The figure shows three views and two pictorial views of one solid part (mm, origin at its lowest corner). Answer the questions. A direction names the side the tool comes from. Round coordinates to 2 decimals unless told otherwise and drop trailing zeros. Order: outer loops, then holes, each group sorted by start corner. A loop starts at its lowest first (then second) coordinate and runs counter-clockwise, first axis right, second up. Notation, with made-up numbers: (36, 68) - (50, 68) arc R15 cw to (50, 94) - close; hole circle Ø8 at (-33, -4.5). An arc over 180 degrees is marked (long way). Use CSV: the item, a comma, the result in double quotes. Start each with the question number.
Item 1: For the marked faces 5, 6 and 7, determine the directions among +Z, -Z, +X, -X, +Y, -Y from which every point of the face is accessible in a straight line to the end or side of a thin tool.
Item 2: Find section D-D, the plane z = 3. Give the vertices of the cut face in (x, y), plus the area to 3 significant figures.
Item 3: Find section A-A, the plane z = 13. Give the vertices of the cut face in (x, y).
Item 4: Straight lines are drawn through the part: line 1 along X through (y, z) = (2.65, 13); line 2 along Z through (x, y) = (10, 1.55); line 3 along X through (y, z) = (3, 7). For each, find the intervals that lie inside material, in ascending order. Write a range as [from, to].
Item 5: Find section C-C, the plane y = 6. Give the vertices of the cut face in (x, z).
Item 6: Flat-ended cylindrical pins translate along their axes: P1, Ø8, axis at x = 32, y = 37.5, coming from the +Z side; P2, Ø1.5, axis at y = 31, z = 10, coming from the +X side; P3, Ø6, axis at x = 20.5, z = 7.5, coming from the +Y side (1 decimal); P4, Ø1.8, axis at x = 4, z = 13, coming from the -Y side. Find the tip coordinate at first contact, or state that the pin passes through.
Item 7: Determine the mould class of the marked faces 1, 2, 3 and 4 for opening direction Y: +Y half, -Y half, draft (parallel to the pull), parting line (faces both ways), or undercut.
Item 8: Find section B-B, the plane x = 10. Give the vertices of the cut face in (y, z).
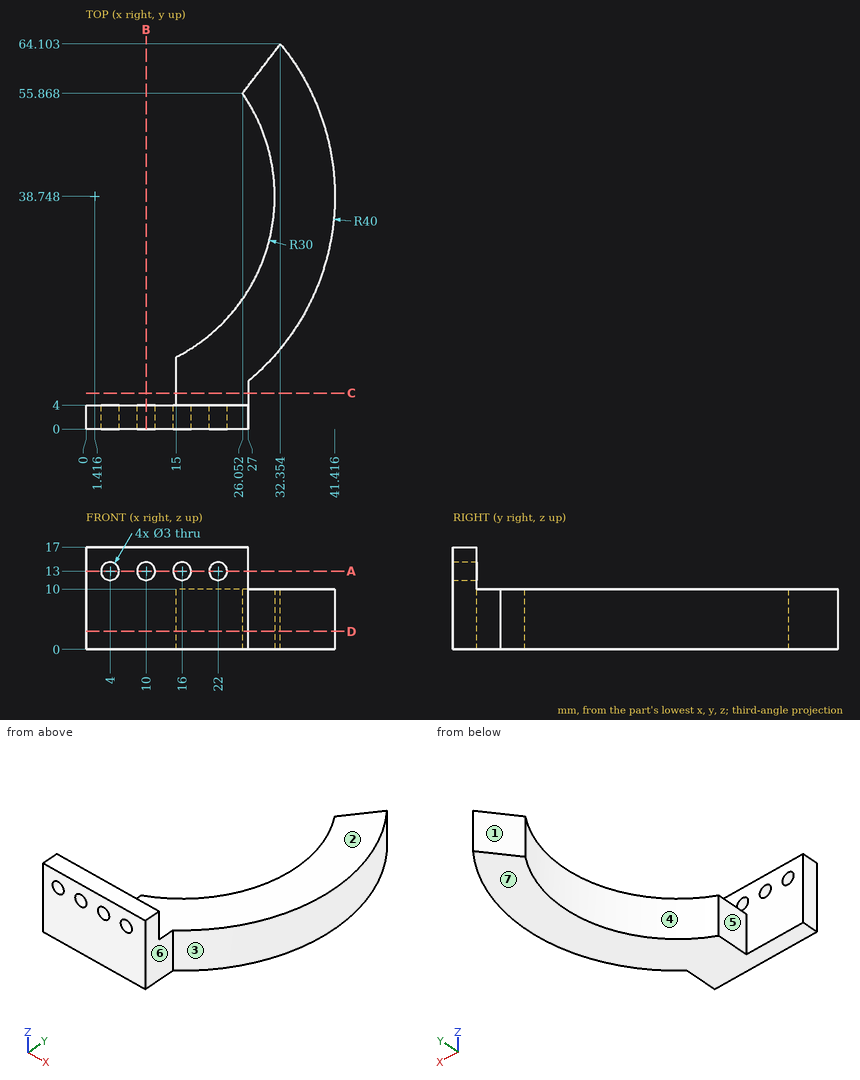
Worked out:
1,face 5,"+Z, -Z, -X, +Y"
1,face 6,"+Z, -Z, +X, -Y"
1,face 7,"-Z, +X, -X, +Y, -Y"
2,outline,"(0, 0) - (27, 0) - (27, 8) arc R40 ccw to (32.35, 64.1) - (26.05, 55.87) arc R30 cw to (15, 12) - (15, 4) - (0, 4) - close"
2,area,"748 mm²"
3,outline,"(0, 0) - (2.5, 0) - (2.5, 4) - (0, 4) - close; (5.5, 0) - (8.5, 0) - (8.5, 4) - (5.5, 4) - close; (11.5, 0) - (14.5, 0) - (14.5, 4) - (11.5, 4) - close; (17.5, 0) - (20.5, 0) - (20.5, 4) - (17.5, 4) - close; (23.5, 0) - (27, 0) - (27, 4) - (23.5, 4) - close"
4,line 1,"x = [0, 2.5], [5.5, 8.5], [11.5, 14.5], [17.5, 20.5], [23.5, 27]"
4,line 2,"z = [0, 11.5], [14.5, 17]"
4,line 3,"x = [0, 27]"
5,outline,"(15, 0) - (27, 0) - (27, 10) - (15, 10) - close"
6,P1,"stops at z = 10"
6,P2,"stops at x = 40.8"
6,P3,"stops at y = 18.4"
6,P4,"passes through"
7,face 1,"+Y half"
7,face 2,"draft"
7,face 3,"parting line"
7,face 4,"undercut"
8,outline,"(0, 0) - (4, 0) - (4, 11.5) - (0, 11.5) - close; (0, 14.5) - (4, 14.5) - (4, 17) - (0, 17) - close"
